from build123d import *

# Parameters (mm, degrees)
SKETCH1_W           = 50
SKETCH1_H           = 171.6
SKETCH1_R           = 2
BOSS_EXTRUDE1_DEPTH = 37.5
CUT_EXTRUDE4_START  = -5
SKETCH2_W           = 50
SKETCH2_H           = 39
SKETCH2_R           = 6
SKETCH2_R_2         = 1.25
CUT_EXTRUDE4_DEPTH  = 30
SKETCH2_3_R         = 1.25
SKETCH2_3_R_2       = 6
CUT_EXTRUDE5_DEPTH  = 178.419869237


with BuildPart() as part:
    # Sketch1 → Boss-Extrude1 (new body)
    with BuildSketch(Plane(origin=(0, 0, 0), x_dir=(1, 0, 0), z_dir=(0, 1, 0))):
        with Locations((0, 85.8)):
            Rectangle(SKETCH1_W, SKETCH1_H)
        with Locations(Location((0, 148.9, 0), (0, 0, 270))):
            Circle(SKETCH1_R, mode=Mode.SUBTRACT)
        with Locations(Location((0, 161.6, 0), (0, 0, 270))):
            Circle(SKETCH1_R, mode=Mode.SUBTRACT)
        with Locations(Location((0, 137.47, 0), (0, 0, 270))):
            Circle(SKETCH1_R, mode=Mode.SUBTRACT)
        with Locations(Location((0, 52.888, 0), (0, 0, 270))):
            Circle(SKETCH1_R, mode=Mode.SUBTRACT)
        with Locations(Location((0, 65.588, 0), (0, 0, 270))):
            Circle(SKETCH1_R, mode=Mode.SUBTRACT)
        with Locations(Location((0, 41.458, 0), (0, 0, 270))):
            Circle(SKETCH1_R, mode=Mode.SUBTRACT)
    extrude(amount=BOSS_EXTRUDE1_DEPTH)

    # Sketch2 → Cut-Extrude4 (cut)
    with BuildSketch(Plane.XZ.offset(CUT_EXTRUDE4_START)):
        with Locations((0, -19.5)):
            Rectangle(SKETCH2_W, SKETCH2_H)
        with Locations(Location((0, -13, 0), (0, 0, 270))):
            Circle(SKETCH2_R, mode=Mode.SUBTRACT)
        with Locations(Location((-15.5, -20, 0), (0, 0, 270))):
            Circle(SKETCH2_R_2, mode=Mode.SUBTRACT)
        with Locations(Location((-7.75, -6.576606241, 0), (0, 0, 270))):
            Circle(SKETCH2_R_2, mode=Mode.SUBTRACT)
        with Locations(Location((7.75, -6.576606241, 0), (0, 0, 270))):
            Circle(SKETCH2_R_2, mode=Mode.SUBTRACT)
        with Locations(Location((15.5, -20, 0), (0, 0, 270))):
            Circle(SKETCH2_R_2, mode=Mode.SUBTRACT)
        with Locations(Location((7.75, -33.423393759, 0), (0, 0, 270))):
            Circle(SKETCH2_R_2, mode=Mode.SUBTRACT)
        with Locations(Location((-7.75, -33.423393759, 0), (0, 0, 270))):
            Circle(SKETCH2_R_2, mode=Mode.SUBTRACT)
    extrude(amount=-CUT_EXTRUDE4_DEPTH, mode=Mode.SUBTRACT)

    # Sketch2_3 → Cut-Extrude5 (cut, through all)
    with BuildSketch(Plane.XZ):
        with Locations(Location((-7.75, -33.423393759, 0), (0, 0, 270))):
            Circle(SKETCH2_3_R)
        with Locations(Location((7.75, -33.423393759, 0), (0, 0, 270))):
            Circle(SKETCH2_3_R)
        with Locations(Location((0, -13, 0), (0, 0, 270))):
            Circle(SKETCH2_3_R_2)
        with Locations(Location((-7.75, -6.576606241, 0), (0, 0, 270))):
            Circle(SKETCH2_3_R)
        with Locations(Location((7.75, -6.576606241, 0), (0, 0, 270))):
            Circle(SKETCH2_3_R)
        with Locations(Location((-15.5, -20, 0), (0, 0, 270))):
            Circle(SKETCH2_3_R)
        with Locations(Location((15.5, -20, 0), (0, 0, 270))):
            Circle(SKETCH2_3_R)
    extrude(amount=-CUT_EXTRUDE5_DEPTH, mode=Mode.SUBTRACT)


solid = part.part
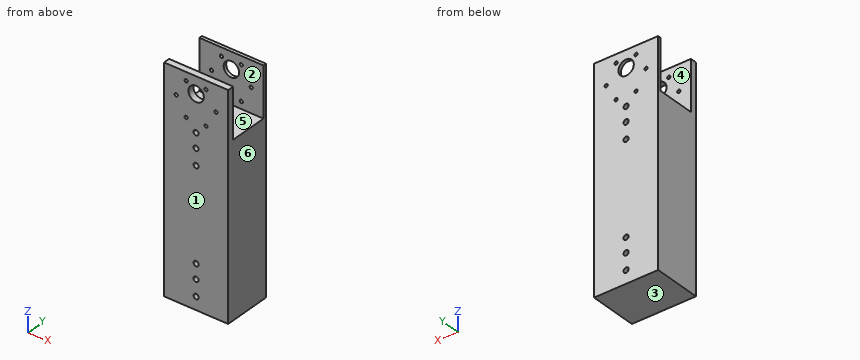
Design review of the part built by this model. Coordinates are the model's own, in mm. Face numbers are marked on the shaded views. A direction names the side the tool comes from. Coordinates: 2 decimals unless noted, no trailing zeros. Loops run counter-clockwise (first coordinate to the right, second up) from the corner with the lowest first, then second, coordinate; pieces in that order, holes last. Notation, with made-up numbers: (42, 0) -> (83, 0) arc R11 cw to (83, 5) -> close; hole circle Ø11 at (49, 27). An arc over 180 degrees is marked (long way). Use a Markdown table: item, result. Add a question column.
Item 1: We need section C-C, the plane z = -10. Write out the cut boundary in (x, y).
Item 2: We need section B-B, the plane y = 29. Write out the cut boundary in (x, z), and give its area (3 significant figures).
Item 3: We need section A-A, the plane z = -148.9. Write out the cut boundary in (x, y), and give its area (4 significant figures).
Item 4: Wall thickness on L1, parallel to X at y = 36.7, z = -13; L2, parallel to Z at x = 7, y = 2; L3, parallel to Y at x = 9, z = -28: over which ranges is each line inside the solid? List them lowest first. Write a range as from..to.
Item 5: We need section D-D, the plane x = 3.5. Write out the cut boundary in (y, z).
Item 6: Clearance check with a flat-ended pin moving along its axis: P1, Ø5, axis at x = -14, y = 16, coming from the +Z side. State where the tip first meets the part, or that it passes through.
Item 7: Machinability: for the marked faces 5 and 6, which of the approach directions +Z, -Z, +X, -X, +Y, -Y give a long, thin tool a straight path to every point of the face, cutting with its end or side? Answer none if there is none.
Item 8: The part is to be moulded in two halves that separate along Y. For the marked faces 1, 2, 3 and 4, say which applies: +Y half, -Y half, draft (parallel to the pull), parting line (faces both ways), or undercut.
Numbers:
| question | item | result |
|---|---|---|
| 1 | outline | (-25, 0) -> (-5.2, 0) -> (-5.2, 5) -> (-25, 5) -> close; (-25, 35) -> (-5.2, 35) -> (-5.2, 37.5) -> (-25, 37.5) -> close; (5.2, 0) -> (25, 0) -> (25, 5) -> (5.2, 5) -> close; (5.2, 35) -> (25, 35) -> (25, 37.5) -> (5.2, 37.5) -> close |
| 2 | outline | (-25, -171.6) -> (25, -171.6) -> (25, -39) -> (-25, -39) -> close; hole circle Ø4 at (0, -161.6); hole circle Ø4 at (0, -148.9); hole circle Ø4 at (0, -137.47); hole circle Ø4 at (0, -65.59); hole circle Ø4 at (0, -52.89); hole circle Ø4 at (0, -41.46) |
| 2 | area | 6,550 mm^2 |
| 3 | outline | (-25, 0) -> (-2, 0) -> (-2, 37.5) -> (-25, 37.5) -> close; (2, 0) -> (25, 0) -> (25, 37.5) -> (2, 37.5) -> close |
| 3 | area | 1,725 mm^2 |
| 4 | L1 | x = -25..-6, 6..25 |
| 4 | L2 | z = -171.6..-34.42, -32.42..-7.58, -5.58..0 |
| 4 | L3 | y = 0..5, 35..37.5 |
| 5 | outline | (0, -171.6) -> (37.5, -171.6) -> (37.5, -17.87) -> (35, -17.87) -> (35, -39) -> (5, -39) -> (5, -17.87) -> (0, -17.87) -> close; (0, -8.13) -> (5, -8.13) -> (5, 0) -> (0, 0) -> close; (35, -8.13) -> (37.5, -8.13) -> (37.5, 0) -> (35, 0) -> close |
| 6 | P1 | stops at z = -39 |
| 7 | face 5 | +Z, +X, -X |
| 7 | face 6 | +Z, -Z, +X, +Y, -Y |
| 8 | face 1 | -Y half |
| 8 | face 2 | undercut |
| 8 | face 3 | draft |
| 8 | face 4 | undercut |
